Can you work these out from the model? Positions are in its coordinate system, mm. A direction names the side the tool comes from. Round coordinates to 2 decimals unless told otherwise and drop trailing zeros. Write each loop counter-clockwise with the first axis right and the second up, starting at its lowest first coordinate (ties: lowest second). Pieces come first, ordered by that corner, then holes. Notation, with made-up numbers: M -17.75,66.25 L 27.25,66.25 A10 ccw 27.25,70.25 Z; hole C 2.5,21.25 d1. An arc over 180 degrees is marked long. Answer in a Markdown table with one row per item. Add a question column.
(1) I'm going to push flat-ended pins straight in: pin 1 (1.9 mm diameter, centred on x = 0, y = -0.5, fed in from +Z); pin 2 (1.7 mm diameter, centred on x = -0.5, z = 3.5, fed in from +Y). Where does each tip first touch, or does it pass through?
(2) If I drill on probe 1 along Z at (x, y) = (1.05, -1.5); probe 2 along Y at (x, z) = (1.3, 4.75), over which ranges is the centre line in solid material (lowest first)?
(3) Suppose I cut it at A-A, the plane x = 0.1. Write out the boundary of the cut face in (y, z), then the cut area to 3 significant figures.
(4) For faces 1 (the face through (0, 0, 1.947)), 2 (the face through (0, -7, 5.403)), which set-ups out of +Z, -Z, +X, -X, +Y, -Y let a thin tool reach every point of the face, with its end or its side?
(5) Suppose I cut it at C-C, the plane z = 4.25. Write out the boundary of the cut face in (x, y), then the cut area to 3 significant figures.
(6) Suppose I cut it at B-B, the plane y = 3.5. Write out the boundary of the cut face in (x, z).
from build123d import *

# Parameters (mm, degrees)
F0_W          = 3.886314
F0_H          = 3.89309
F1_DEPTH      = 5.08
F1_DEPTH_BACK = 5.08
F2_W          = 3.886314
F2_H          = 7.349639
F3_DEPTH      = 3.81


with BuildPart() as f1:
    # F0 (on Front) → F1 (new body, two sides)
    with BuildSketch(Plane.XZ) as f1_sk:
        Rectangle(F0_W, F0_H)
    extrude(amount=F1_DEPTH)
    extrude(f1_sk.sketch, amount=-F1_DEPTH_BACK)

    # F2 (on face) → F3 (join)
    with BuildSketch(Plane.XZ.offset(5.08)):
        with Locations((0, 1.728274)):
            Rectangle(F2_W, F2_H)
    extrude(amount=F3_DEPTH)


solid = f1.part
Calculated:
| question | item | result |
|---|---|---|
| 1 | pin 1 | z = 1.95 |
| 1 | pin 2 | y = -5.08 |
| 2 | probe 1 | -1.95 to 1.95 |
| 2 | probe 2 | -8.89 to -5.08 |
| 3 | outline | M -8.89,-1.95 L 5.08,-1.95 L 5.08,1.95 L -5.08,1.95 L -5.08,5.4 L -8.89,5.4 Z |
| 3 | area | 67.6 mm² |
| 4 | face 1 | +Z, +X, -X, +Y |
| 4 | face 2 | +Z, +X, -X, +Y, -Y |
| 5 | outline | M -1.94,-8.89 L 1.94,-8.89 L 1.94,-5.08 L -1.94,-5.08 Z |
| 5 | area | 14.8 mm² |
| 6 | outline | M -1.94,-1.95 L 1.94,-1.95 L 1.94,1.95 L -1.94,1.95 Z |
